The model under review builds one solid part; all positions refer to its coordinate system, in mm. A direction names the side the tool comes from. Give positions to 0.01 mm unless a question says otherwise; leave off trailing zeros. Write each loop counter-clockwise with the first axis right and the second up, starting at its lowest first coordinate (ties: lowest second). Pieces come first, ordered by that corner, then holes. Notation, with made-up numbers: M 50,13.5 L 96,13.5 A17 ccw 96,32.5 Z; hole C 34.25,47 d1. An arc over 180 degrees is marked long. Write each question's results on one line, items separated by ' | '. Start each with the question number.
from build123d import *

# Parameters (mm, degrees)
F0_R     = 13.2
F0_R_2   = 11.2
F1_DEPTH = 7


with BuildPart() as f1:
    # F0 (on Top) → F1 (new body)
    with BuildSketch(Plane.XY):
        with BuildLine():
            ThreePointArc((11.632991, 20.493819), (-0.73006, 13.552093), (-12.250791, 21.816798))
            Line((-12.250791, 21.816798), (-12.596717, 21.818154))
            Line((-12.596717, 21.818154), (-12.623499, 14.987107))
            Line((-12.623499, 14.987107), (-17.952998, 15.692942))
            Line((-17.952998, 15.692942), (-14.466907, 9.654855))
            Line((-14.466907, 9.654855), (-20.082159, 8.081509))
            Line((-20.082159, 8.081509), (-17.656412, 3.77544))
            Line((-17.656412, 3.77544), (-23.564664, -0.172444))
            ThreePointArc((-23.564664, -0.172444), (-13.964283, -3.886835), (-9.950495, -13.365945))
            ThreePointArc((-9.950495, -13.365945), (-10.674874, -17.678585), (-12.768506, -21.517895))
            Line((-12.768506, -21.517895), (-12.596717, -21.818154))
            Line((-12.596717, -21.818154), (-6.667466, -18.425824))
            Line((-6.667466, -18.425824), (-4.613987, -23.394224))
            Line((-4.613987, -23.394224), (-1.127896, -17.356137))
            Line((-1.127896, -17.356137), (3.042287, -21.432415))
            Line((3.042287, -21.432415), (5.558579, -17.178622))
            Line((5.558579, -17.178622), (11.931673, -20.321376))
            ThreePointArc((11.931673, -20.321376), (12.324979, -5.812918), (25.805954, -0.435804))
            Line((25.805954, -0.435804), (25.193434, 0))
            Line((25.193434, 0), (19.290965, 3.438717))
            Line((19.290965, 3.438717), (22.566986, 7.701282))
            Line((22.566986, 7.701282), (15.594803, 7.701282))
            Line((15.594803, 7.701282), (17.039872, 13.350905))
            Line((17.039872, 13.350905), (12.097833, 13.403182))
            Line((12.097833, 13.403182), (11.632991, 20.493819))
        make_face()
        Circle(F0_R, mode=Mode.SUBTRACT)
        Circle(F0_R)
        Circle(F0_R_2, mode=Mode.SUBTRACT)
        with BuildLine():
            ThreePointArc((36.350495, -13.365945), (33.380159, -5.023644), (25.805954, -0.435804))
            ThreePointArc((25.805954, -0.435804), (12.324979, -5.812918), (11.931673, -20.321376))
            ThreePointArc((11.931673, -20.321376), (26.766539, -26.060992), (36.350495, -13.365945))
        make_face()
        with Locations((23.150495, -13.365945)):
            Circle(F0_R_2, mode=Mode.SUBTRACT)
        with BuildLine():
            ThreePointArc((-9.950495, -13.365945), (-13.964283, -3.886835), (-23.564664, -0.172444))
            ThreePointArc((-23.564664, -0.172444), (-34.929563, -19.323592), (-12.768506, -21.517895))
            ThreePointArc((-12.768506, -21.517895), (-10.674874, -17.678585), (-9.950495, -13.365945))
        make_face()
        with Locations((-23.150495, -13.365945)):
            Circle(F0_R_2, mode=Mode.SUBTRACT)
        with BuildLine():
            ThreePointArc((11.632991, 20.493819), (12.802255, 23.515951), (13.2, 26.731889))
            ThreePointArc((13.2, 26.731889), (-2.502954, 39.692414), (-12.250791, 21.816798))
            ThreePointArc((-12.250791, 21.816798), (-0.73006, 13.552093), (11.632991, 20.493819))
        make_face()
        with Locations((0, 26.731889)):
            Circle(F0_R_2, mode=Mode.SUBTRACT)
    extrude(amount=F1_DEPTH)


solid = f1.part
(1) Draft analysis for pull direction X (two halves, no side actions). For faces 6 (the flat face through (16.31, 10.49, 3.45)), 7 (the flat face through (8.701, -18.728, 3.451)), 8 (the flat face through (0.93, -19.37, 3.45)), 9 (the flat face through (19, 7.701, 3)), state which applies: pulls with the +X half, pulls with the -X half, needs draft (parallel to the pull), parting line crosses it, or undercut.
(2) Clearance check with flat-ended pins moving along their axes: P1, Ø3, axis at y = -3, z = 4, coming from the -X side; P2, Ø6, axis at x = -7.5, y = 26.5, coming from the -Z side. State where each tip first meets the part, or that it passes through.
(3) Add section A-A (z = 2). Give the number of separate pieces and of enclosed holes in the cut face, then the cut area to 3 significant figures.
(4) Add section D-D (x = 7). State the section outline as (y, z) points.
(5) Wall thickness on L1, parallel to X at y = -17, z = 6.75; L2, parallel to Y at x = 0, z = 5.5; L3, parallel to Y at x = -0.5, z = 0.5: over which ranges is each line inside the solid? List them lowest first.
(6) Machinability: for faces 1 (the flat face through (20.906, 5.54, 3.451)), 2 (the flat face through (-9.674, -20.146, 3.451)), 3 (the flat face through (-17.235, 8.879, 3.451)), 4 (the flat face through (5.2, -10.4, 0)), 5 (the cylindrical face through (6.021, 36.176, 3.451)), which of the approach directions +Z, -Z, +X, -X, +Y, -Y give a long, thin tool a straight path to every point of the face, cutting with its end or side? Answer none if there is none.
(7) Add section C-C (y = -3). State the section outline as (x, z) points, then the cut area to 3 significant figures.
(8) Add section B-B (x = 28.5). State the section outline as (y, z) points, then the cut area to 3 significant figures.
Calculated:
1) face 6: pulls with the +X half | face 7: undercut | face 8: undercut | face 9: needs draft
2) P1: stops at x = -32.93 | P2: passes through
3) separate pieces: 1 | enclosed holes: 4 | area: 1,110 mm²
4) outline: M -17.89,0 L -8.74,0 L -8.74,7 L -17.89,7 Z; M 8.74,0 L 17.99,0 L 17.99,7 L 8.74,7 Z; M 35.47,0 L 37.92,0 L 37.92,7 L 35.47,7 Z
5) L1: x = -35.84 to -33.74, -12.56 to 12.56, 33.74 to 35.84 | L2: y = -18.46 to -11.2, 11.2 to 15.53, 37.93 to 39.93 | L3: y = -17.97 to -11.19, 11.19 to 15.54, 37.92 to 39.92
6) face 1: +Z, -Z, +X | face 2: +Z, -Z, -Y | face 3: +Z, -Z, -X | face 4: -Z, +X, -X, +Y, -Y | face 5: +Z, -Z
7) outline: M -31.32,0 L -27.39,0 L -27.39,7 L -31.32,7 Z; M -18.91,0 L -10.79,0 L -10.79,7 L -18.91,7 Z; M 10.79,0 L 18.91,0 L 18.91,7 L 10.79,7 Z; M 27.39,0 L 31.32,0 L 31.32,7 L 27.39,7 Z | area: 169 mm²
8) outline: M -25.43,0 L -23.21,0 L -23.21,7 L -25.43,7 Z; M -3.53,0 L -1.3,0 L -1.3,7 L -3.53,7 Z | area: 31.2 mm²
